CAD build for the part. Positions are in the model's coordinates, mm. Round coordinates to 2 decimals unless told otherwise and drop trailing zeros. Loops run counter-clockwise (first coordinate to the right, second up) from the corner with the lowest first, then second, coordinate; pieces in that order, holes last.
from build123d import *

# Parameters (mm, degrees)
F0_R         = 2
F0_R_2       = 3
F0_R_3       = 11
F1_DEPTH     = 3
F2_T4_DEPTH  = 52.9473251324
F3_T4_DEPTH  = 48.8454257103
F4_T4_DEPTH  = 56.77883553
F4_T10_DEPTH = 56.77883553
F4_T15_DEPTH = 52.9473251324
F4_T20_DEPTH = 52.9473251324
F4_T25_DEPTH = 56.77883553
F4_T31_DEPTH = 56.77883553
F4_T36_DEPTH = 52.9473251324
F4_T41_DEPTH = 52.9473251324
F4_T47_DEPTH = 52.9473251324
F4_T51_DEPTH = 52.9473251324
F4_T58_DEPTH = 52.9473251324
F4_T62_DEPTH = 52.9473251324


# Not quite as in the source:
# - a fillet or chamfer that OpenCascade refuses, or shapes differently, is made with other operations: its cross-section is extruded or revolved along the edge and cut away or added


with BuildPart() as f1:
    # F0 (on Top) → F1 (new body)
    with BuildSketch(Plane.XY):
        Polygon((-14.1421356237, 14.1421356237), (-50, 0), (-14.1421356237, -14.1421356237), (0, -50), (14.1421356237, -14.1421356237), (50, 0), (14.1421356237, 14.1421356237), (0, 50), align=None)
        with Locations((-4.1164257564, -30)):
            Circle(F0_R, mode=Mode.SUBTRACT)
        with Locations((-30, -4.0949434042)):
            Circle(F0_R, mode=Mode.SUBTRACT)
        with Locations((0, -40)):
            Circle(F0_R, mode=Mode.SUBTRACT)
        with Locations((4.0949434042, -30)):
            Circle(F0_R, mode=Mode.SUBTRACT)
        with Locations((0, -20)):
            Circle(F0_R_2, mode=Mode.SUBTRACT)
        with Locations((30, -4.1164257564)):
            Circle(F0_R, mode=Mode.SUBTRACT)
        with Locations((-40, 0)):
            Circle(F0_R, mode=Mode.SUBTRACT)
        with Locations((-30, 4.1164257564)):
            Circle(F0_R, mode=Mode.SUBTRACT)
        with Locations((-20, 0)):
            Circle(F0_R_2, mode=Mode.SUBTRACT)
        with Locations((-4.0949434042, 30)):
            Circle(F0_R, mode=Mode.SUBTRACT)
        Circle(F0_R_3, mode=Mode.SUBTRACT)
        with Locations((20, 0)):
            Circle(F0_R_2, mode=Mode.SUBTRACT)
        with Locations((0, 20)):
            Circle(F0_R_2, mode=Mode.SUBTRACT)
        with Locations((30, 4.0949434042)):
            Circle(F0_R, mode=Mode.SUBTRACT)
        with Locations((40, 0)):
            Circle(F0_R, mode=Mode.SUBTRACT)
        with Locations((4.1164257564, 30)):
            Circle(F0_R, mode=Mode.SUBTRACT)
        with Locations((0, 40)):
            Circle(F0_R, mode=Mode.SUBTRACT)
    extrude(amount=F1_DEPTH)

    # F2: chamfer of 2.8 on 1 edges, made by hand


with BuildPart() as f2_tool2:
    # F2_s3 → F2_t4 (new body)
    with BuildSketch(Plane(origin=(-19.7071398503, -49.9681212794, 0), x_dir=(0, 0, 1), z_dir=(0.3668907842, 0.930264023, 0))):
        Polygon((0.2, 18.3445392079), (3, 15.5445392079), (3, 18.3445392079), align=None)
    extrude(amount=F2_T4_DEPTH)

    split(bisect_by=Plane(origin=(6.730442375, -17.0652648437, 0), x_dir=(0, 0, 1), z_dir=(0.3668907842, -0.930264023, 0)), keep=Keep.TOP)


with BuildPart() as f1_1:
    add(f1.part)

    # F2_t1: cut F2_tool2
    add(f2_tool2.part, mode=Mode.SUBTRACT)

    # F3: chamfer of 2.8 on 1 edges, made by hand


with BuildPart() as f3_tool2:
    # F3_s3 → F3_t4 (new body)
    with BuildSketch(Plane(origin=(0.2812542134, -0.7131295943, 0), x_dir=(0, 0, 1), z_dir=(0.3668907842, -0.930264023, 0))):
        Polygon((3, 15.5445392079), (0.2, 18.3445392079), (3, 18.3445392079), align=None)
    extrude(amount=F3_T4_DEPTH)

    split(bisect_by=Plane(origin=(-6.730442375, -17.0652648437, 0), x_dir=(0, 0, 1), z_dir=(-0.3668907842, -0.930264023, 0)), keep=Keep.TOP)


with BuildPart() as f1_2:
    add(f1_1.part)

    # F3_t1: cut F3_tool2
    add(f3_tool2.part, mode=Mode.SUBTRACT)

    # F4: chamfer of 2.8 on 6 edges, made by hand


with BuildPart() as f4_tool2:
    # F4_s3 → F4_t4 (new body)
    with BuildSketch(Plane(origin=(-2.8511866823, -1.1244916409, 0), x_dir=(0, 0, 1), z_dir=(0.930264023, 0.3668907842, 0))):
        Polygon((3, 15.5445392079), (0.2, 18.3445392079), (3, 18.3445392079), align=None)
    extrude(amount=F4_T4_DEPTH)

    split(bisect_by=Plane(origin=(17.0652648437, -6.730442375, 0), x_dir=(0, 0, 1), z_dir=(-0.930264023, 0.3668907842, 0)), keep=Keep.TOP)

    split(bisect_by=Plane(origin=(8.6256588242, -3.4019102659, 9.272269604), x_dir=(0.3668907842, 0.930264023, 0), z_dir=(0.657795999, -0.2594309614, 0.7071067812)), keep=Keep.TOP)


with BuildPart() as f1_3:
    add(f1_2.part)

    # F4_t1: cut F4_tool2
    add(f4_tool2.part, mode=Mode.SUBTRACT)


with BuildPart() as f4_tool8:
    # F4_s9 → F4_t10 (new body)
    with BuildSketch(Plane(origin=(-2.8511866823, -1.1244916409, 0), x_dir=(0, 0, 1), z_dir=(0.930264023, 0.3668907842, 0))):
        Polygon((3, 15.5445392079), (0.2, 18.3445392079), (3, 18.3445392079), align=None)
    extrude(amount=F4_T10_DEPTH)

    split(bisect_by=Plane(origin=(17.0652648437, -6.730442375, 0), x_dir=(0, 0, 1), z_dir=(0.930264023, -0.3668907842, 0)), keep=Keep.TOP)


with BuildPart() as f1_4:
    add(f1_3.part)

    # F4_t7: cut F4_tool8
    add(f4_tool8.part, mode=Mode.SUBTRACT)


with BuildPart() as f4_tool13:
    # F4_s14 → F4_t15 (new body)
    with BuildSketch(Plane(origin=(49.9681212794, -19.7071398503, 0), x_dir=(0, 0, 1), z_dir=(-0.930264023, 0.3668907842, 0))):
        Polygon((3, 15.5445392079), (0.2, 18.3445392079), (3, 18.3445392079), align=None)
    extrude(amount=F4_T15_DEPTH)

    split(bisect_by=Plane(origin=(17.0652648437, 6.730442375, 0), x_dir=(0, 0, 1), z_dir=(0.930264023, 0.3668907842, 0)), keep=Keep.TOP)


with BuildPart() as f1_5:
    add(f1_4.part)

    # F4_t12: cut F4_tool13
    add(f4_tool13.part, mode=Mode.SUBTRACT)


with BuildPart() as f4_tool18:
    # F4_s19 → F4_t20 (new body)
    with BuildSketch(Plane(origin=(-0.2812542134, 0.7131295943, 0), x_dir=(0, 0, 1), z_dir=(-0.3668907842, 0.930264023, 0))):
        Polygon((3, 15.5445392079), (0.2, 18.3445392079), (3, 18.3445392079), align=None)
    extrude(amount=F4_T20_DEPTH)

    split(bisect_by=Plane(origin=(6.730442375, 17.0652648437, 0), x_dir=(0, 0, 1), z_dir=(0.3668907842, 0.930264023, 0)), keep=Keep.TOP)


with BuildPart() as f1_6:
    add(f1_5.part)

    # F4_t17: cut F4_tool18
    add(f4_tool18.part, mode=Mode.SUBTRACT)


with BuildPart() as f4_tool23:
    # F4_s24 → F4_t25 (new body)
    with BuildSketch(Plane(origin=(2.8511866823, -1.1244916409, 0), x_dir=(0, 0, 1), z_dir=(-0.930264023, 0.3668907842, 0))):
        Polygon((3, -15.5445392079), (0.2, -18.3445392079), (3, -18.3445392079), align=None)
    extrude(amount=F4_T25_DEPTH)

    split(bisect_by=Plane(origin=(-17.0652648437, -6.730442375, 0), x_dir=(0, 0, 1), z_dir=(0.930264023, 0.3668907842, 0)), keep=Keep.TOP)

    split(bisect_by=Plane(origin=(-8.6256588242, -3.4019102659, 9.272269604), x_dir=(0.3668907842, -0.930264023, 0), z_dir=(-0.657795999, -0.2594309614, 0.7071067812)), keep=Keep.TOP)


with BuildPart() as f1_7:
    add(f1_6.part)

    # F4_t22: cut F4_tool23
    add(f4_tool23.part, mode=Mode.SUBTRACT)


with BuildPart() as f4_tool29:
    # F4_s30 → F4_t31 (new body)
    with BuildSketch(Plane(origin=(2.8511866823, -1.1244916409, 0), x_dir=(0, 0, 1), z_dir=(-0.930264023, 0.3668907842, 0))):
        Polygon((3, -15.5445392079), (0.2, -18.3445392079), (3, -18.3445392079), align=None)
    extrude(amount=F4_T31_DEPTH)

    split(bisect_by=Plane(origin=(-17.0652648437, -6.730442375, 0), x_dir=(0, 0, 1), z_dir=(-0.930264023, -0.3668907842, 0)), keep=Keep.TOP)


with BuildPart() as f1_8:
    add(f1_7.part)

    # F4_t28: cut F4_tool29
    add(f4_tool29.part, mode=Mode.SUBTRACT)


with BuildPart() as f4_tool34:
    # F4_s35 → F4_t36 (new body)
    with BuildSketch(Plane(origin=(-0.7131295943, -0.2812542134, 0), x_dir=(0, 0, 1), z_dir=(-0.930264023, -0.3668907842, 0))):
        Polygon((0.2, 18.3445392079), (3, 15.5445392079), (3, 18.3445392079), align=None)
    extrude(amount=F4_T36_DEPTH)

    split(bisect_by=Plane(origin=(-17.0652648437, 6.730442375, 0), x_dir=(0, 0, 1), z_dir=(-0.930264023, 0.3668907842, 0)), keep=Keep.TOP)


with BuildPart() as f1_9:
    add(f1_8.part)

    # F4_t33: cut F4_tool34
    add(f4_tool34.part, mode=Mode.SUBTRACT)


with BuildPart() as f4_tool39:
    # F4_s40 → F4_t41 (new body)
    with BuildSketch(Plane(origin=(19.7071398503, 49.9681212794, 0), x_dir=(0, 0, 1), z_dir=(-0.3668907842, -0.930264023, 0))):
        Polygon((3, 15.5445392079), (0.2, 18.3445392079), (3, 18.3445392079), align=None)
    extrude(amount=F4_T41_DEPTH)

    split(bisect_by=Plane(origin=(-6.730442375, 17.0652648437, 0), x_dir=(0, 0, 1), z_dir=(-0.3668907842, 0.930264023, 0)), keep=Keep.TOP)


with BuildPart() as f1_10:
    add(f1_9.part)

    # F4_t38: cut F4_tool39
    add(f4_tool39.part, mode=Mode.SUBTRACT)


with BuildPart() as f4_tool45:
    # F4_s46 → F4_t47 (new body)
    with BuildSketch(Plane(origin=(-0.2812542134, 0.7131295943, 0), x_dir=(0, 0, 1), z_dir=(-0.3668907842, 0.930264023, 0))):
        Polygon((3, 15.5445392079), (0.2, 18.3445392079), (3, 18.3445392079), align=None)
    extrude(amount=F4_T47_DEPTH)

    split(bisect_by=Plane(origin=(6.730442375, 17.0652648437, 0), x_dir=(0, 0, 1), z_dir=(-0.3668907842, -0.930264023, 0)), keep=Keep.TOP)


with BuildPart() as f4_tool49:
    # F4_s50 → F4_t51 (new body)
    with BuildSketch(Plane(origin=(49.9681212794, -19.7071398503, 0), x_dir=(0, 0, 1), z_dir=(-0.930264023, 0.3668907842, 0))):
        Polygon((3, 15.5445392079), (0.2, 18.3445392079), (3, 18.3445392079), align=None)
    extrude(amount=F4_T51_DEPTH)

    split(bisect_by=Plane(origin=(17.0652648437, 6.730442375, 0), x_dir=(0, 0, 1), z_dir=(-0.930264023, -0.3668907842, 0)), keep=Keep.TOP)


with BuildPart() as f4_tool45_1:
    add(f4_tool45.part)

    # F4_t53: intersect F4_tool49
    add(f4_tool49.part, mode=Mode.INTERSECT)


with BuildPart() as f1_11:
    add(f1_10.part)

    # F4_t43: cut F4_tool45
    add(f4_tool45_1.part, mode=Mode.SUBTRACT)


with BuildPart() as f4_tool56:
    # F4_s57 → F4_t58 (new body)
    with BuildSketch(Plane(origin=(-0.7131295943, -0.2812542134, 0), x_dir=(0, 0, 1), z_dir=(-0.930264023, -0.3668907842, 0))):
        Polygon((0.2, 18.3445392079), (3, 15.5445392079), (3, 18.3445392079), align=None)
    extrude(amount=F4_T58_DEPTH)

    split(bisect_by=Plane(origin=(-17.0652648437, 6.730442375, 0), x_dir=(0, 0, 1), z_dir=(0.930264023, -0.3668907842, 0)), keep=Keep.TOP)


with BuildPart() as f4_tool60:
    # F4_s61 → F4_t62 (new body)
    with BuildSketch(Plane(origin=(19.7071398503, 49.9681212794, 0), x_dir=(0, 0, 1), z_dir=(-0.3668907842, -0.930264023, 0))):
        Polygon((3, 15.5445392079), (0.2, 18.3445392079), (3, 18.3445392079), align=None)
    extrude(amount=F4_T62_DEPTH)

    split(bisect_by=Plane(origin=(-6.730442375, 17.0652648437, 0), x_dir=(0, 0, 1), z_dir=(0.3668907842, -0.930264023, 0)), keep=Keep.TOP)


with BuildPart() as f4_tool56_1:
    add(f4_tool56.part)

    # F4_t64: intersect F4_tool60
    add(f4_tool60.part, mode=Mode.INTERSECT)


with BuildPart() as f1_12:
    add(f1_11.part)

    # F4_t54: cut F4_tool56
    add(f4_tool56_1.part, mode=Mode.SUBTRACT)


solid = f1_12.part
Item 1: Cut at A-A (x = 30). List the corners of the cut face in (y, z), plus the area to 3 significant figures.
Verdict:
outline: (-7.89, 0) - (-6.12, 0) - (-6.12, 1.85) - (-7.89, 0.2) - close; (-2.12, 0) - (2.09, 0) - (2.09, 3) - (-2.12, 3) - close; (6.09, 0) - (7.89, 0) - (7.89, 0.2) - (6.09, 1.87) - close
area: 16.3 mm2
Item 2: Wall check: L1, parallel to X at y = -31, z = 1.2; L2, parallel to X at y = -30, z = 1.35; L3, parallel to X at y = 37.5, z = 2.95. Give the ranges that are in metal, low to high.
Verdict:
L1: x = -6.42 to -5.85, -2.38 to 2.36, 5.83 to 6.42
L2: x = -6.65 to -6.12, -2.12 to 2.09, 6.09 to 6.65
L3: x = -1.97 to 1.97
Item 3: Cut at D-D (y = -20). List the corners of the cut face in (x, z).
Verdict:
outline: (-11.83, 0) - (-3, 0) - (-3, 3) - (-8.82, 3) - (-11.83, 0.2) - close; (3, 0) - (11.83, 0) - (11.83, 0.2) - (8.82, 3) - (3, 3) - close
Item 4: Cut at C-C (z = 0.75). State how many separate pieces and enclosed holes the cut face has, plus the area to 3 significant figures.
Verdict:
separate pieces: 1
enclosed holes: 17
area: 2,020 mm2
Item 5: Mould opens along Y. For faces 1 (the flat face through (30.84, -6.365, 1.308)), 2 (the cylindrical face through (-0.65, -22.93, 1.48)), 3 (the cylindrical face through (-29.08, 2.34, 1.48)), 4 (the flat face through (27.134, 7.492, 1.62)) say: released by +Y, released by -Y, zero draft, split by the parting line, or undercut.
Verdict:
face 1: released by -Y
face 2: undercut
face 3: undercut
face 4: released by +Y
Item 6: Cut at B-B (y = -40). List the corners of the cut face in (x, z), plus the area to 3 significant figures.
Verdict:
outline: (-3.94, 0) - (-2, 0) - (-2, 2.01) - (-3.94, 0.2) - close; (2, 0) - (3.94, 0) - (3.94, 0.2) - (2, 2.01) - close
area: 4.29 mm2
Item 7: Flat gauge pins, fed straight in: P1, Ø1.5, axis at x = -27.5, z = 0.5, coming from the -Y side (3 decimals); P2, Ø1.5, axis at x = -24.5, z = 0.5, coming from the -Y side. Where does each tip first touch, or does it go through?
Verdict:
P1: stops at y = -9.145
P2: stops at y = -10.33
